For this review, take the finished solid that the model builds, in its own axes (mm). A direction names the side the tool comes from. Coordinates: 2 decimals unless noted, no trailing zeros. Loops run counter-clockwise (first coordinate to the right, second up) from the corner with the lowest first, then second, coordinate; pieces in that order, holes last. Notation, with made-up numbers: M -9,43.25 L 43,43.25 A19 cw 43,55.25 Z; hole C 11.5,85 d6. An arc over 180 degrees is marked long. Write item = value, one per line.
from build123d import *

# Parameters (mm, degrees)
F0_R           = 1.5
F1_DEPTH       = 8
F2_D           = 5.2
F2_DEPTH       = 30
F2_CBORE_D     = 10.2
F2_CBORE_DEPTH = 1.5
F2_TIP         = 1.5622376095
F4_D           = 3
F4_DEPTH       = 20
F4_TIP         = 0.9012909285
F5_D           = 3
F5_DEPTH       = 20
F5_CBORE_D     = 5.3
F5_CBORE_DEPTH = 4
F5_TIP         = 0.9012909285


with BuildPart() as f1:
    # F0 (on Top) → F1 (new body)
    with BuildSketch(Plane.XY):
        with BuildLine():
            Line((-21.4485637844, 22.2857501358), (-21.4485637844, 37.2857501358))
            ThreePointArc((-21.4485637844, 37.2857501358), (-32.5263109951, 29.7857501358), (-21.4485637844, 22.2857501358))
        make_face()
        with BuildLine():
            ThreePointArc((-16.3708165737, 29.7857501358), (-17.7596460232, 34.3143679364), (-21.4485637844, 37.2857501358))
            Line((-21.4485637844, 37.2857501358), (-21.4485637844, 22.2857501358))
            ThreePointArc((-21.4485637844, 22.2857501358), (-17.7596460232, 25.2571323352), (-16.3708165737, 29.7857501358))
        make_face()
        with BuildLine():
            Line((-13.4485637844, 22.2857501358), (-13.4485637844, 37.2857501358))
            Line((-13.4485637844, 37.2857501358), (-21.4485637844, 37.2857501358))
            ThreePointArc((-21.4485637844, 37.2857501358), (-17.7596460232, 34.3143679364), (-16.3708165737, 29.7857501358))
            ThreePointArc((-16.3708165737, 29.7857501358), (-17.7596460232, 25.2571323352), (-21.4485637844, 22.2857501358))
            Line((-21.4485637844, 22.2857501358), (-13.4485637844, 22.2857501358))
        make_face()
        with BuildLine():
            Line((6.9514365147, 31.482860446), (6.9514365147, 37.2857501358))
            Line((6.9514365147, 37.2857501358), (-13.4485637844, 37.2857501358))
            Line((-13.4485637844, 37.2857501358), (-13.4485637844, 22.2857501358))
            Line((-13.4485637844, 22.2857501358), (-13.4485637844, -13.1142501633))
            Line((-13.4485637844, -13.1142501633), (-13.4485637844, -28.1142501633))
            Line((-13.4485637844, -28.1142501633), (-13.4485637844, -39.2912365496))
            Line((-13.4485637844, -39.2912365496), (6.9514365147, -39.2912365496))
            Line((6.9514365147, -39.2912365496), (6.9514365147, -28.1142501633))
            Line((6.9514365147, -28.1142501633), (6.9514365147, -2.9142498642))
            ThreePointArc((6.9514365147, -2.9142498642), (4.637909559, 4.5857501358), (6.9514365147, 12.0857501358))
            Line((6.9514365147, 12.0857501358), (6.9514365147, 31.482860446))
        make_face()
        with Locations((-7.7535887534, -32.4602356078)):
            Circle(F0_R, mode=Mode.SUBTRACT)
        Polygon((-1.2058451539, 19.7087634504), (1.1941548461, 19.7087634504), (1.9514365147, 19.7087634504), (1.9514365147, -26.2912365496), (-8.4485637844, -26.2912365496), (-8.4485637844, 19.7087634504), align=None, mode=Mode.SUBTRACT)
        with Locations((0.2464112466, 24.5397643922)):
            Circle(F0_R, mode=Mode.SUBTRACT)
        with BuildLine():
            ThreePointArc((20.9514365147, 29.5776203275), (15.8929462828, 36.9579798621), (6.9514365147, 37.2857501358))
            Line((6.9514365147, 37.2857501358), (6.9514365147, 31.482860446))
            ThreePointArc((6.9514365147, 31.482860446), (11.3811141914, 32.3344336643), (14.9514365147, 29.5776203275))
            Line((14.9514365147, 29.5776203275), (14.9514365147, 12.0857501358))
            ThreePointArc((14.9514365147, 12.0857501358), (17.9514365147, 12.6634973465), (20.9514365147, 12.0857501358))
            Line((20.9514365147, 12.0857501358), (20.9514365147, 26.9164390002))
            Line((20.9514365147, 26.9164390002), (20.9514365147, 29.5776203275))
        make_face()
        with BuildLine():
            Line((20.9514365147, 12.0857501358), (14.9514365147, 12.0857501358))
            Line((14.9514365147, 12.0857501358), (14.9514365147, -2.9142498642))
            ThreePointArc((14.9514365147, -2.9142498642), (22.4800543153, -2.1031676254), (26.0291837254, 4.5857501358))
            ThreePointArc((26.0291837254, 4.5857501358), (24.6403542759, 9.1143679364), (20.9514365147, 12.0857501358))
        make_face()
        with BuildLine():
            ThreePointArc((20.9514365147, 12.0857501358), (17.9514365147, 12.6634973465), (14.9514365147, 12.0857501358))
            Line((14.9514365147, 12.0857501358), (20.9514365147, 12.0857501358))
        make_face()
        with BuildLine():
            Line((14.9514365147, -2.9142498642), (14.9514365147, 12.0857501358))
            ThreePointArc((14.9514365147, 12.0857501358), (9.873689304, 4.5857501358), (14.9514365147, -2.9142498642))
        make_face()
        with BuildLine():
            Line((-13.4485637844, -28.1142501633), (-13.4485637844, -13.1142501633))
            Line((-13.4485637844, -13.1142501633), (-21.4485637844, -13.1142501633))
            ThreePointArc((-21.4485637844, -13.1142501633), (-17.7596460232, -16.0856323627), (-16.3708165737, -20.6142501633))
            ThreePointArc((-16.3708165737, -20.6142501633), (-17.7596460232, -25.1428679639), (-21.4485637844, -28.1142501633))
            Line((-21.4485637844, -28.1142501633), (-13.4485637844, -28.1142501633))
        make_face()
        with BuildLine():
            ThreePointArc((-16.3708165737, -20.6142501633), (-17.7596460232, -16.0856323627), (-21.4485637844, -13.1142501633))
            Line((-21.4485637844, -13.1142501633), (-21.4485637844, -28.1142501633))
            ThreePointArc((-21.4485637844, -28.1142501633), (-17.7596460232, -25.1428679639), (-16.3708165737, -20.6142501633))
        make_face()
        with BuildLine():
            Line((-21.4485637844, -28.1142501633), (-21.4485637844, -13.1142501633))
            ThreePointArc((-21.4485637844, -13.1142501633), (-32.5263109951, -20.6142501633), (-21.4485637844, -28.1142501633))
        make_face()
    extrude(amount=F1_DEPTH)

    # F2
    with Locations(Plane(origin=(0, 0, 0), x_dir=(1, 0, 0), z_dir=(0, 0, -1))):
        with Locations((17.9514365147, -4.5857501358), (-24.4485637844, -29.7857501358), (-24.4485637844, 20.6142501633)):
            CounterBoreHole(F2_D / 2, F2_CBORE_D / 2, F2_CBORE_DEPTH, depth=F2_DEPTH)
            with Locations((0, 0, -(F2_DEPTH + F2_TIP / 2))):  # 118° drill point
                Cone(0, F2_D / 2, F2_TIP, mode=Mode.SUBTRACT)

    # F4
    with Locations(Plane.YZ.offset(20.9514365147)):
        with Locations((16.0857501358, 4)):
            Hole(F4_D / 2, depth=F4_DEPTH)
            with Locations((0, 0, -(F4_DEPTH + F4_TIP / 2))):  # 118° drill point
                Cone(0, F4_D / 2, F4_TIP, mode=Mode.SUBTRACT)

    # F5
    with Locations(Plane(origin=(0, 0, 0), x_dir=(1, 0, 0), z_dir=(0, 0, -1))):
        with Locations((0.2464112466, -24.5397643922), (-7.7535887534, 32.4602356078)):
            CounterBoreHole(F5_D / 2, F5_CBORE_D / 2, F5_CBORE_DEPTH, depth=F5_DEPTH)
            with Locations((0, 0, -(F5_DEPTH + F5_TIP / 2))):  # 118° drill point
                Cone(0, F5_D / 2, F5_TIP, mode=Mode.SUBTRACT)


solid = f1.part
Q1. Machinability: for faces 1 (the face through (6.951, 22, 4)), 2 (the face through (-3, 19.709, 4)), 3 (the face through (-9.71, -34.25, 1.97)), 4 (the face through (16, 36.9, 3.9)), which of the approach directions +Z, -Z, +X, -X, +Y, -Y give a long, thin tool a straight path to every point of the face, cutting with its end or side? Answer none if there is none.
Solved:
face_1 = +Z, -Z, -Y
face_2 = +Z, -Z
face_3 = -Z
face_4 = +Z, -Z, +Y
Q2. Draft analysis for pull direction X (two halves, no side actions). For faces 5 (the face through (-28.21, -24.06, 0.74)), 6 (the face through (4.416, 15.279, 5.265)), state which applies: +X half, -X half, draft (parallel to the pull), parting line (faces both ways), or undercut.
Solved:
face_5 = undercut
face_6 = draft
Q3. Add section B-B (y = -24). Write out the cut boundary in (x, z).
Solved:
outline = M -31.78,0 L -28.26,0 L -28.26,1.5 L -20.63,1.5 L -20.63,0 L -8.45,0 L -8.45,8 L -31.78,8 Z; M 1.95,0 L 6.95,0 L 6.95,8 L 1.95,8 Z
Q4. Add section A-A (x = -17). Write out the cut boundary in (y, z), and give its area (3 significant figures).
Solved:
outline = M -28.11,0 L -13.11,0 L -13.11,8 L -28.11,8 Z; M 22.29,0 L 37.29,0 L 37.29,8 L 22.29,8 Z
area = 240 mm²
Q5. For line 1 along X through (y, z) = (17.5, 4.75); line 2 along X through (y, z) = (-9, 6.5); line 3 along Y through (x, z) = (-17.5, 3.75), list the stretches that pass through material, from the lowest coordinate up.
Solved:
line_1 = -13.45 to -8.45, 1.95 to 6.95, 14.95 to 20.95
line_2 = -13.45 to -8.45, 1.95 to 6.95
line_3 = -28.11 to -13.11, 22.29 to 37.29
Q6. For pin 1 Ø3 at (x, y) = (-26.5, -20.5) entering from -Z; pin 2 Ø4 at (y, z) = (22.5, 4) entering from -X; pin 3 Ø3.5 at (y, z) = (16.09, 4) entering from +X, all flat-tipped, find the tip position at first contact; note any pin that passes through.
Solved:
pin_1 = 1.5
pin_2 = -30.56
pin_3 = 20.95
